from build123d import *

# Parameters (mm, degrees)
F_10_0_1935_DIAMETER_HOLE1_D = 4.9149
CIRPATTERN3_COUNT            = 6
CUT_EXTRUDE1_DEPTH           = 13.7
FILLET1_R                    = 4
CIRPATTERN4_COUNT            = 6
FILLET1_OF_CIRPATTERN4_R     = 4
CHAMFER1_SIZE                = 1
CHAMFER2_SIZE                = 1


with BuildPart() as part:
    # Sketch2 → Revolve1 (revolve)
    with BuildSketch(Plane(origin=(0, 0, 0), x_dir=(0, 0, -1), z_dir=(1, 0, 0))):
        Polygon((-39.2125, 0), (-82.55, 0), (-82.55, 12.7), (-49.2125, 12.7), (-49.2125, 10), (-39.2125, 10), align=None)
    revolve(axis=Axis((0, -0.635, 0), (0, 1, 0)))

    # #10 (0.1935) Diameter Hole1 (through all)
    with Locations(Plane(origin=(0, 12.7, 0), x_dir=(1, 0, 0), z_dir=(0, 1, 0))):
        with Locations((-35, 60.621778)):
            f_10_0_1935_diameter_hole1 = Hole(F_10_0_1935_DIAMETER_HOLE1_D / 2)

    # CirPattern3: #10 (0.1935) Diameter Hole1 ×6 about axis
    cirpattern3_axis = Axis((0, 0, 0), (0, 1, 0))
    for i in range(1, CIRPATTERN3_COUNT):
        add(f_10_0_1935_diameter_hole1.rotate(cirpattern3_axis, i * 360 / CIRPATTERN3_COUNT), mode=Mode.SUBTRACT)

    # Sketch8 → Cut-Extrude1 (cut, through all)
    with BuildSketch(Plane(origin=(0, 12.7, 0), x_dir=(1, 0, 0), z_dir=(0, 1, 0))):
        with BuildLine():
            Line((-34.364196, 69.520533), (-22.66059, 49.249293))
            ThreePointArc((-22.66059, 49.249293), (0, 54.2125), (22.66059, 49.249293))
            Line((22.66059, 49.249293), (34.364196, 69.520533))
            ThreePointArc((34.364196, 69.520533), (0, 77.55), (-34.364196, 69.520533))
        make_face()
    cut_extrude1 = extrude(amount=-CUT_EXTRUDE1_DEPTH, mode=Mode.SUBTRACT)

    # Fillet1
    fillet1_edges = [part.edges().sort_by_distance(p)[0] for p in [
        (22.66059, 6.35, -49.249293),
        (-22.66059, 6.35, -49.249293),
        (-34.364196, 6.35, -69.520533),
        (34.364196, 6.35, -69.520533),
    ]]
    fillet(fillet1_edges, radius=FILLET1_R)

    # CirPattern4: Cut-Extrude1 ×6 about axis
    cirpattern4_axis = Axis((0, 0, 0), (0, 1, 0))
    for i in range(1, CIRPATTERN4_COUNT):
        add(cut_extrude1.rotate(cirpattern4_axis, i * 360 / CIRPATTERN4_COUNT), mode=Mode.SUBTRACT)

    # Fillet1 of CirPattern4
    fillet1_of_cirpattern4_edges = [part.edges().sort_by_distance(p)[0] for p in [
        (-31.320844, 6.35, -44.249293),
        (-53.981433, 6.35, -5),
        (-77.388646, 6.35, -5),
        (-43.02445, 6.35, -64.520533),
        (-53.981433, 6.35, 5),
        (-31.320844, 6.35, 44.249293),
        (-43.02445, 6.35, 64.520533),
        (-77.388646, 6.35, 5),
        (-22.66059, 6.35, 49.249293),
        (22.66059, 6.35, 49.249293),
        (34.364196, 6.35, 69.520533),
        (-34.364196, 6.35, 69.520533),
        (31.320844, 6.35, 44.249293),
        (53.981433, 6.35, 5),
        (77.388646, 6.35, 5),
        (43.02445, 6.35, 64.520533),
        (53.981433, 6.35, -5),
        (31.320844, 6.35, -44.249293),
        (43.02445, 6.35, -64.520533),
        (77.388646, 6.35, -5),
    ]]
    fillet(fillet1_of_cirpattern4_edges, radius=FILLET1_OF_CIRPATTERN4_R)

    # Chamfer1
    chamfer1_edges = [part.edges().sort_by_distance(p)[0] for p in [
        (0, 12.7, -49.2125),
    ]]
    chamfer(chamfer1_edges, length=CHAMFER1_SIZE)

    # Chamfer2
    chamfer2_edges = [part.edges().sort_by_distance(p)[0] for p in [
        (0, 0, -82.55),
    ]]
    chamfer(chamfer2_edges, length=CHAMFER2_SIZE)


solid = part.part
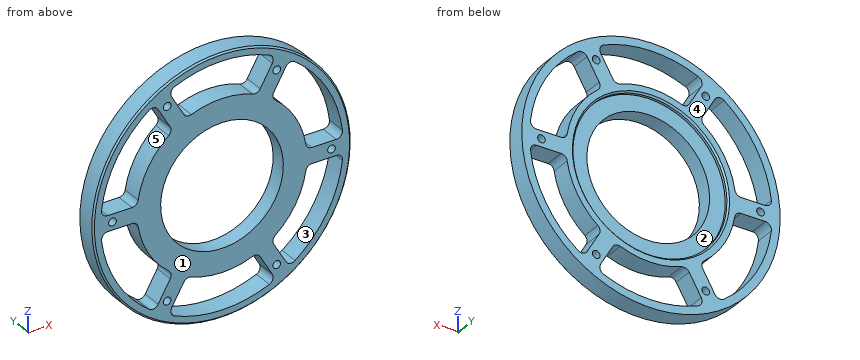
Geometry: final body of the model. Coordinates: model frame, mm. Face numbers are marked on the shaded views. A direction names the side the tool comes from. Give positions to 0.01 mm unless a question says otherwise; leave off trailing zeros. Write each loop counter-clockwise with the first axis right and the second up, starting at its lowest first coordinate (ties: lowest second). Pieces come first, ordered by that corner, then holes.
(1) Cut plane B-B, the plane x = 0. Return loops of the section in (y, z).
(2) Access query for the marked faces 1 and 2. Directions: +Z, -Z, +X, -X, +Y, -Y. A direction counts if a zero-diameter tool reaches every point of the face in a straight line with its end or side. Return the directions, or none.
(3) Ray query, line 1 (Z direction, x = -39.5, y = 11.5); line 2 (Z direction, x = -64.5, y = 6.5); line 3 (Z direction, x = -55, y = 6). Return the intervals inside material, ascending.
(4) Mould query, pull axis Z, two halves, no side actions, for the marked faces 3, 4 and 5. Classes: released by +Z, released by -Z, zero draft, split by the parting line, or undercut.
(5) Cut plane C-C, the plane y = 3.5. Give the number of separate pieces and of enclosed holes in the cut face, then the cut area to 3 significant figures.
(6) Cut plane A-A, the plane z = 0. Return loops of the section in (x, y), then the cut area to 3 significant figures.
(7) First-contact query: P1, Ø4, axis at y = 2.5, z = -11, coming from the +X side; P2, Ø5, axis at y = 6.5, z = 45, coming from the +X side; P3, Ø6.5, axis at x = -70, z = 0, coming from the -Y side; P4, Ø2, axis at y = 10.5, z = -3.5, coming from the -X side. Flat tips, straight axial feed; report the tip coordinate or a pass-through.
Values follow:
1. outline: (0, -81.55) - (1, -82.55) - (12.7, -82.55) - (12.7, -77.55) - (0, -77.55) - close; (0, -54.21) - (12.7, -54.21) - (12.7, -50.21) - (11.7, -49.21) - (10, -49.21) - (10, -39.21) - (0, -39.21) - close; (0, 39.21) - (10, 39.21) - (10, 49.21) - (11.7, 49.21) - (12.7, 50.21) - (12.7, 54.21) - (0, 54.21) - close; (0, 77.55) - (12.7, 77.55) - (12.7, 82.55) - (1, 82.55) - (0, 81.55) - close
2. face 1: +Z, -Z, +X, -X, -Y
2. face 2: +Y
3. line 1: z = -72.49 to -58.42, -37.13 to -29.35, 29.35 to 37.13, 58.42 to 72.49
3. line 2: z = -51.52 to -43.06, -5 to 5, 43.06 to 51.52
3. line 3: z = -61.56 to -54.67, -5.89 to 5.89, 54.67 to 61.56
4. face 3: undercut
4. face 4: zero draft
4. face 5: undercut
5. separate pieces: 1
5. enclosed holes: 13
5. area: 8,290 mm2
6. outline: (-82.55, 1) - (-81.55, 0) - (-72.46, 0) - (-72.46, 12.7) - (-82.55, 12.7) - close; (-67.54, 0) - (-39.21, 0) - (-39.21, 10) - (-49.21, 10) - (-49.21, 11.7) - (-50.21, 12.7) - (-67.54, 12.7) - close; (39.21, 0) - (67.54, 0) - (67.54, 12.7) - (50.21, 12.7) - (49.21, 11.7) - (49.21, 10) - (39.21, 10) - close; (72.46, 0) - (81.55, 0) - (82.55, 1) - (82.55, 12.7) - (72.46, 12.7) - close
6. area: 920 mm2
7. P1: stops at x = 82.06
7. P2: stops at x = 70.77
7. P3: stops at y = 0
7. P4: stops at x = -82.51
